Autodesk Inventor part; units mm, degrees
ref_plane "YZ Plane" through (0, 0, 0) normal (1, 0, 0) x (0, 1, 0)
ref_plane "XZ Plane" through (0, 0, 0) normal (0, 1, 0) x (-1, 0, 0)
ref_plane "XY Plane" through (0, 0, 0) normal (0, 0, 1) x (1, 0, 0)
sketch "tabs" plane through (0, 0, 0) normal (0, 0, 1) x (1, 0, 0)
  line L0 (15.6175, 13.9118) -> (18.7675, 13.9118)
  line L1 (18.7675, 13.9118) -> (18.7675, 10.7868)
  line L2 (18.7675, 10.7868) -> (15.6175, 10.7868)
  line L3 (15.6175, 10.7868) -> (15.6175, 13.9118)
  line L4 (21.8175, 13.9118) -> (24.9675, 13.9118)
  line L5 (24.9675, 13.9118) -> (24.9675, 10.7868)
  line L6 (24.9675, 10.7868) -> (21.8175, 10.7868)
  line L7 (21.8175, 10.7868) -> (21.8175, 13.9118)
  line L8 (28.0175, 13.9118) -> (31.1675, 13.9118)
  line L9 (31.1675, 13.9118) -> (31.1675, 10.7868)
  line L10 (31.1675, 10.7868) -> (28.0175, 10.7868)
  line L11 (28.0175, 10.7868) -> (28.0175, 13.9118)
  line L12 (23.3925, 10.7868) -> (23.3925, 8.8536) construction
  point P0 (23.3925, 12.1901)
  dimension "d2" = 3.15
  dimension "d3" = 3.05
  dimension "d4" = 3.05
  dimension "d5" = 3.125
sketch "Sketch1" plane through (0, 0, 0) normal (0, 0, 1) x (1, 0, 0)
  line L0 (-6, 20) -> (6, 20)
  line L1 (16, 10) -> (16, 0)
  line L2 (16, 0) -> (-16, 0)
  line L3 (-16, 0) -> (-16, 10)
  line L4 (0, 16.9043) -> (0, -20.0235) construction
  line L5 (-32.3473, 0) -> (40.4078, 0) construction
  arc A0 (-6, 20) -> (-16, 10) centre (-6, 10) ccw
  arc A1 (16, 10) -> (6, 20) centre (6, 10) ccw
  circle A2 centre (0, 14) radius 1.5
  line L6 (-7.775, 0) -> (-4.625, 0)
  line L7 (-4.625, 0) -> (-4.625, -3.125)
  line L8 (-4.625, -3.125) -> (-7.775, -3.125)
  line L9 (-7.775, -3.125) -> (-7.775, 0)
  line L10 (-1.575, 0) -> (1.575, 0)
  line L11 (1.575, 0) -> (1.575, -3.125)
  line L12 (1.575, -3.125) -> (-1.575, -3.125)
  line L13 (-1.575, -3.125) -> (-1.575, 0)
  line L14 (4.625, 0) -> (7.775, 0)
  line L15 (7.775, 0) -> (7.775, -3.125)
  line L16 (7.775, -3.125) -> (4.625, -3.125)
  line L17 (4.625, -3.125) -> (4.625, 0)
  line L18 (0, -3.125) -> (0, -5.0582) construction
  point P0 (0, 0)
  point P1 (0, 20)
  point P2 (16, 5)
  dimension "d0" = 32
  dimension "d6" = 20
  dimension "d7" = 10
  dimension "d8" = 3
  dimension "d9" = 6
extrude "Extrusion1" add sketch "Sketch1" along normal blind 3.1
equation "\"d2\" = mat + kerf"
equation "\"d3\" = mat - kerf"
equation "\"d4\" = mat - kerf"
equation "\"d5\" = mat + 0.5 * kerf"
equation "\"d10\" = mat"
properties part number "link1"
Geometry: final body of the model. Coordinates: model frame, mm. A direction names the side the tool comes from. Give positions to 0.01 mm unless a question says otherwise; leave off trailing zeros. Write each loop counter-clockwise with the first axis right and the second up, starting at its lowest first coordinate (ties: lowest second). Pieces come first, ordered by that corner, then holes. Notation, with made-up numbers: (22.25, 50.5) -> (31.25, 50.5) arc R21 ccw to (31.25, 79.5) -> close; hole circle Ø4 at (29.25, -27.75). An arc over 180 degrees is marked (long way). Answer as a JSON object with one key per item and string values.
1. Access query for faces 5 (the flat face through (-6, -3.125, 2)), 6 (the flat face through (-12, 0, 2)), 7 (the flat face through (-4.625, -2, 2)), 8 (the flat face through (12, 0, 2)). Directions: +Z, -Z, +X, -X, +Y, -Y. A direction counts if a zero-diameter tool reaches every point of the face in a straight line with its end or side. Return the directions, or none.
Ans:
{"face 5": "+Z, -Z, +X, -X, -Y", "face 6": "+Z, -Z, -X, -Y", "face 7": "+Z, -Z, -Y", "face 8": "+Z, -Z, +X, -Y"}
2. Cut plane B-B on x = 0. Output: boundary loops of the cut face in (y, z) (3 decimals).
Ans:
{"outline": "(-3.125, 0) -> (12.5, 0) -> (12.5, 3.1) -> (-3.125, 3.1) -> close; (15.5, 0) -> (20, 0) -> (20, 3.1) -> (15.5, 3.1) -> close"}
3. Cut plane C-C on y = -0.75. Output: boundary loops of the cut face in (x, z) (3 decimals).
Ans:
{"outline": "(-7.775, 0) -> (-4.625, 0) -> (-4.625, 3.1) -> (-7.775, 3.1) -> close; (-1.575, 0) -> (1.575, 0) -> (1.575, 3.1) -> (-1.575, 3.1) -> close; (4.625, 0) -> (7.775, 0) -> (7.775, 3.1) -> (4.625, 3.1) -> close"}
4. Contact query for flat-ended pins moving along their axis: pin 1 (0.9 mm diameter, centred on y = -1, z = 1.5, fed in from -X) (3 decimals); pin 2 (1.6 mm diameter, centred on x = 11.5, z = 1.5, fed in from -Y); pin 3 (1.6 mm diameter, centred on y = -2.5, z = 1, fed in from +X) (3 decimals). Output: stop coordinate, or through.
Ans:
{"pin 1": "stops at x = -7.775", "pin 2": "stops at y = 0", "pin 3": "stops at x = 7.775"}
5. Cut plane A-A on z = 1.6. Output: boundary loops of the cut face in (x, y) (3 decimals), and give its area (3 significant figures).
Ans:
{"outline": "(-16, 0) -> (-7.775, 0) -> (-7.775, -3.125) -> (-4.625, -3.125) -> (-4.625, 0) -> (-1.575, 0) -> (-1.575, -3.125) -> (1.575, -3.125) -> (1.575, 0) -> (4.625, 0) -> (4.625, -3.125) -> (7.775, -3.125) -> (7.775, 0) -> (16, 0) -> (16, 10) arc R10 ccw to (6, 20) -> (-6, 20) arc R10 ccw to (-16, 10) -> close; hole circle Ø3 at (0, 14)", "area": "620 mm^2"}
6. Ray query, probe 1 along X at (y, z) = (-1.25, 2.7) (3 decimals); probe 2 along Y at (x, z) = (0, 1.9) (3 decimals); probe 3 along X at (y, z) = (14.75, 1.2). Return the intervals inside material, ascending. Write a range as from..to.
Ans:
{"probe 1": "x = -7.775..-4.625, -1.575..1.575, 4.625..7.775", "probe 2": "y = -3.125..12.5, 15.5..20", "probe 3": "x = -14.8..-1.3, 1.3..14.8"}
7. Cut plane D-D on y = 13. Output: boundary loops of the cut face in (x, z), and give its area (3 significant figures).
Ans:
{"outline": "(-15.54, 0) -> (-1.12, 0) -> (-1.12, 3.1) -> (-15.54, 3.1) -> close; (1.12, 0) -> (15.54, 0) -> (15.54, 3.1) -> (1.12, 3.1) -> close", "area": "89.4 mm^2"}
8. Mould query, pull axis X, two halves, no side actions, for faces 1 (the flat face through (16, 5, 2)), 2 (the flat face through (0, 20, 2)), 3 (the cylindrical face through (-13.15, 16.99, 1.53)), 4 (the flat face through (-3, 0, 2)). Classes: pulls with the +X half, pulls with the -X half, needs draft (parallel to the pull), parting line crosses it, or undercut.
Ans:
{"face 1": "pulls with the +X half", "face 2": "needs draft", "face 3": "pulls with the -X half", "face 4": "undercut"}
